Input: part model. Units: mm. Frame: model coordinates. A direction names the side the tool comes from. Round coordinates to 2 decimals unless told otherwise and drop trailing zeros. Loops run counter-clockwise (first coordinate to the right, second up) from the corner with the lowest first, then second, coordinate; pieces in that order, holes last. Notation, with made-up numbers: (64.5, -25.5) -> (106.5, -25.5) arc R27 cw to (106.5, -6.5) -> close; hole circle Ø2 at (65.5, -10.75). An arc over 180 degrees is marked (long way). Answer in a Markdown table with one row per item. Add a question column.
Q1. Section C-C, the plane y = 27. Output: boundary loops of the cut face in (x, z), and give its area (3 significant figures).
Q2. Section B-B, the plane y = 35. Output: boundary loops of the cut face in (x, z), and give its area (3 significant figures).
Q3. Section D-D, the plane y = 41. Output: boundary loops of the cut face in (x, z).
Q4. Ray query, L1, parallel to Z at x = -1, y = 34; L2, parallel to X at y = 42.25, z = 0 (3 decimals); L3, parallel to Z at x = 0, y = 42. Return the intervals inside material, ascending. Write a range as from..to.
Q5. Reachability of faces 1 (the face through (-9.76, 38.87, -2.17)), 2 (the face through (0, 0, 0)) from +Z, -Z, +X, -X, +Y, -Y: full face, straight path, thin tool, end or side. Return the list, or none.
Q6. Section A-A, the plane x = 0. Output: boundary loops of the cut face in (y, z).
Q7. Mould query, pull axis Z, two halves, no side actions, for faces 3 (the face through (3, 50, 12)), 4 (the face through (16.544, 26.549, -5.21)), 5 (the face through (0, 30, 0)). Classes: pulls with the +Z half, pulls with the -Z half, needs draft (parallel to the pull), parting line crosses it, or undercut.
Q8. Pin query (flat end, axial travel): pin 1 (16 mm diameter, centred on x = -2, z = -3, fed in from +Y); pin 2 (1.5 mm diameter, centred on y = 22.5, z = -6, fed in from +X); pin 3 (2 mm diameter, centred on x = 5.5, y = 36, fed in from +Z). Return the tip coordinate at first contact, or that it passes through.
```python
from build123d import *

# Parameters (mm, degrees)
SKETCH2_R               = 15
SKETCH1_R               = 20
CUT_EXTRUDE1_DEPTH      = 58.445626622
CUT_EXTRUDE1_DEPTH_BACK = 20
SKETCH3_R               = 10
FILLET1_R               = 5
FILLET2_R               = 2


with BuildPart() as part:
    # Sketch2 → Loft1 section 0
    with BuildSketch(Plane(origin=(0, 50, 0), x_dir=(1, 0, 0), z_dir=(0, 1, 0))):
        Circle(SKETCH2_R)
    # Sketch1 → Loft1 section 1
    with BuildSketch(Plane(origin=(0, 0, 0), x_dir=(1, 0, 0), z_dir=(0, 1, 0))):
        Circle(SKETCH1_R)
    loft()

    # Sketch3 → Cut-Extrude1 (cut, two sides: drawn at the far end of the back side and taken through both)
    with BuildSketch(Plane(origin=(0, 50, 0), x_dir=(1, 0, 0), z_dir=(0, 1, 0)).offset(-CUT_EXTRUDE1_DEPTH_BACK)):
        with Locations(Location((0, 0, 0), (0, 0, 270))):
            Circle(SKETCH3_R)
    extrude(amount=CUT_EXTRUDE1_DEPTH + CUT_EXTRUDE1_DEPTH_BACK, mode=Mode.SUBTRACT)

    # Fillet1
    fillet1_edges = [part.edges().sort_by_distance(p)[0] for p in [
        (-20, 0, 0),
    ]]
    fillet(fillet1_edges, radius=FILLET1_R)

    # Fillet2
    fillet2_edges = [part.edges().sort_by_distance(p)[0] for p in [
        (-15, 50, 0),
        (0, 50, -10),
    ]]
    fillet(fillet2_edges, radius=FILLET2_R)


solid = part.part
```
Answer block:
| question | item | result |
|---|---|---|
| 1 | outline | circle Ø34.6 at (0, 0) |
| 1 | area | 940 mm^2 |
| 2 | outline | circle Ø33 at (0, 0); hole circle Ø20 at (0, 0) |
| 2 | area | 541 mm^2 |
| 3 | outline | circle Ø31.8 at (0, 0); hole circle Ø20 at (0, 0) |
| 4 | L1 | -16.57..-9.95, 9.95..16.57 |
| 4 | L2 | -15.775..-10, 10..15.775 |
| 4 | L3 | -15.8..-10, 10..15.8 |
| 5 | face 1 | +Y |
| 5 | face 2 | +Z, -Z, +X, -X, -Y |
| 6 | outline | (0, -14.48) arc R5 ccw to (5.5, -19.45) -> (48.2, -15.18) arc R2 ccw to (50, -13.19) -> (50, -12) arc R2 ccw to (48, -10) -> (30, -10) -> (30, 10) -> (48, 10) arc R2 ccw to (50, 12) -> (50, 13.19) arc R2 ccw to (48.2, 15.18) -> (5.5, 19.45) arc R5 ccw to (0, 14.48) -> close |
| 7 | face 3 | needs draft |
| 7 | face 4 | parting line crosses it |
| 7 | face 5 | undercut |
| 8 | pin 1 | y = 49.96 |
| 8 | pin 2 | x = 16.97 |
| 8 | pin 3 | z = 15.79 |
